Source: CAD feature listing. Evaluate the final solid. Frame: model axes, mm. A direction names the side the tool comes from. Round coordinates to 2 decimals unless told otherwise and drop trailing zeros. Order: outer loops, then holes, each group sorted by start corner. A loop starts at its lowest first (then second) coordinate and runs counter-clockwise, first axis right, second up. Notation, with made-up numbers: (-11.75, 31.25) - (21.25, 31.25) arc R34 cw to (21.25, 67.25) - close; hole circle Ø10 at (-12.5, 63). An arc over 180 degrees is marked (long way). Put each result on its own line as item: value. Start each with the question number.
1) Section B-B on y = 3.5. State how many separate pieces and enclosed holes the cut face has, then the cut area to 3 significant figures.
2) Section A-A on y = 1.9. Output: boundary loops of the cut face in (x, z), then the cut area to 3 significant figures.
3) Line query: probe 1 along X at (y, z) = (1.8, 0); probe 2 along Y at (x, z) = (-1, 6); probe 3 along Z at (x, y) = (-3.75, 5.5). Output: solid intervals per line, ascending. Write a range as [from, to].
4) Access query for faces 1 (the face through (0, 8, 0)), 2 (the face through (-3, 3, 0)). Directions: +Z, -Z, +X, -X, +Y, -Y. A direction counts if a zero-diameter tool reaches every point of the face in a straight line with its end or side. Return the directions, or none.
5) Contact query for flat-ended pins moving along their axis: P1, Ø2, axis at x = 4.5, y = 7, coming from the +Z side; P2, Ø3, axis at x = 5, z = 0.5, coming from the +Y side; P3, Ø2.5, axis at x = 4.5, z = 0, coming from the +Y side. Output: stop coordinate, or through.
6) Mould query, pull axis Z, two halves, no side actions, for faces 3 (the face through (-4, 0.2, 0)), 4 (the face through (0, 0.2, 0)). Classes: +Z half, -Z half, draft (parallel to the pull), parting line (faces both ways), or undercut.
```python
from build123d import *

# Parameters (mm, degrees)
ESQUISSE1_R             = 8
ESQUISSE1_R_2           = 1.5
BOSS_EXTRU_1_DEPTH      = 8
ESQUISSE2_R             = 3
ENL_V_MAT_EXTRU_1_DEPTH = 3
ESQUISSE3_R             = 2
ENL_V_MAT_EXTRU_2_DEPTH = 20
CONG_1_R                = 5
ESQUISSE4_R             = 8
BOSS_EXTRU_2_DEPTH      = 0.2


with BuildPart() as part:
    # Esquisse1 → Boss.-Extru.1 (new body)
    with BuildSketch(Plane(origin=(0, 0, 0), x_dir=(1, 0, 0), z_dir=(0, 1, 0))):
        with Locations(Location((0, 0, 0), (0, 0, 270))):
            Circle(ESQUISSE1_R)
        with Locations(Location((-4.5, 0, 0), (0, 0, 270))):
            Circle(ESQUISSE1_R_2, mode=Mode.SUBTRACT)
        with Locations(Location((4.5, 0, 0), (0, 0, 90))):
            Circle(ESQUISSE1_R_2, mode=Mode.SUBTRACT)
    extrude(amount=BOSS_EXTRU_1_DEPTH)

    # Esquisse2 → Enlèv. mat.-Extru.1 (cut)
    with BuildSketch(Plane(origin=(0, 8, 0), x_dir=(1, 0, 0), z_dir=(0, 1, 0))):
        with Locations(Location((-4.5, 0, 0), (0, 0, 270))):
            Circle(ESQUISSE2_R)
        with Locations(Location((4.5, 0, 0), (0, 0, 270))):
            Circle(ESQUISSE2_R)
    extrude(amount=-ENL_V_MAT_EXTRU_1_DEPTH, mode=Mode.SUBTRACT)

    # Esquisse3 → Enlèv. mat.-Extru.2 (cut, symmetric)
    with BuildSketch(Plane.XY):
        with Locations((0, 1.9)):
            Circle(ESQUISSE3_R)
    extrude(amount=ENL_V_MAT_EXTRU_2_DEPTH, both=True, mode=Mode.SUBTRACT)

    # Congé1
    # the kernel refuses this fillet: 5 mm, written as the material it takes off along each edge
    with BuildSketch(Plane(origin=(0, 8, 0), x_dir=(0, 0, 1), z_dir=(-1, 0, 0))) as cong_1_piece_1:
        with BuildLine():
            CenterArc((8 - CONG_1_R, -CONG_1_R), CONG_1_R, 0, 90)
            Line((8 - CONG_1_R, 0), (8, 0))
            Line((8, 0), (8, -CONG_1_R))
        make_face()
    revolve(axis=Axis((0, 8, 0), (0, 1, 0)), mode=Mode.SUBTRACT)

    # Esquisse4 → Boss.-Extru.2 (add)
    with BuildSketch(Plane.XZ):
        with Locations(Location((0, 0, 0), (0, 0, 262.432428308))):
            Circle(ESQUISSE4_R)
    extrude(amount=-BOSS_EXTRU_2_DEPTH)


solid = part.part
```
Answer sheet:
1. separate pieces: 2
1. enclosed holes: 2
1. area: 148 mm^2
2. outline: (-2, -7.75) - (-2, 7.75) arc R8 ccw to start; (2, -7.75) arc R8 ccw to (2, 7.75) - close; hole circle Ø3 at (-4.5, 0); hole circle Ø3 at (4.5, 0)
2. area: 124 mm^2
3. probe 1: [-8, -6], [-3, -2], [2, 3], [6, 8]
3. probe 2: [0, 0.2], [3.63, 6.94]
3. probe 3: [-6.3, -2.9], [2.9, 6.3]
4. face 1: +Z, -Z, +X, -X, +Y
4. face 2: +Y
5. P1: z = 5.62
5. P2: y = 5
5. P3: y = 0.2
6. face 3: undercut
6. face 4: draft
